For this review, take the finished solid that the model builds, in its own axes (mm). A direction names the side the tool comes from. Round coordinates to 2 decimals unless told otherwise and drop trailing zeros. Order: outer loops, then holes, each group sorted by start corner. A loop starts at its lowest first (then second) coordinate and runs counter-clockwise, first axis right, second up. Notation, with made-up numbers: M 25.25,21.5 L 76.25,21.5 A23 ccw 76.25,33.5 Z; hole C 34,61 d3. An arc over 180 degrees is marked long. Answer as a JSON object with one key per item and string values.
from build123d import *

# Parameters (mm, degrees)
SKETCH1_W                 = 71
SKETCH1_H                 = 250
BOSS_EXTRUDE1_DEPTH       = 5
SKETCH2_W                 = 65
SKETCH2_H                 = 45
BOSS_EXTRUDE3_DEPTH       = 2
LPATTERN1_COUNT           = 5
LPATTERN1_PITCH           = 50
SKETCH3_W                 = 69
SKETCH3_H                 = 48.754858224
BOSS_EXTRUDE8_DEPTH       = 25
LPATTERN5_COUNT           = 5
LPATTERN5_PITCH           = 50
LPATTERN6_COUNT           = 2
LPATTERN6_PITCH           = 70
LPATTERN6_COPY_1_SKETCH_W = 65
LPATTERN6_COPY_1_SKETCH_H = 45
LPATTERN6_COPY_1_DEPTH    = 2
LPATTERN6_COPY_2_SKETCH_W = 65
LPATTERN6_COPY_2_SKETCH_H = 45
LPATTERN6_COPY_2_DEPTH    = 2
LPATTERN6_COPY_3_SKETCH_W = 65
LPATTERN6_COPY_3_SKETCH_H = 45
LPATTERN6_COPY_3_DEPTH    = 2
LPATTERN6_COPY_4_SKETCH_W = 65
LPATTERN6_COPY_4_SKETCH_H = 45
LPATTERN6_COPY_4_DEPTH    = 2
LPATTERN6_COPY_5_SKETCH_W = 69
LPATTERN6_COPY_5_SKETCH_H = 48.754858224
LPATTERN6_COPY_5_DEPTH    = 25
LPATTERN6_COPY_6_SKETCH_W = 69
LPATTERN6_COPY_6_SKETCH_H = 48.754858224
LPATTERN6_COPY_6_DEPTH    = 25
LPATTERN6_COPY_7_SKETCH_W = 69
LPATTERN6_COPY_7_SKETCH_H = 48.754858224
LPATTERN6_COPY_7_DEPTH    = 25
LPATTERN6_COPY_8_SKETCH_W = 69
LPATTERN6_COPY_8_SKETCH_H = 48.754858224
LPATTERN6_COPY_8_DEPTH    = 25


with BuildPart() as part:
    # Sketch1 → Boss-Extrude1 (new body)
    with BuildSketch(Plane(origin=(0, 0, 0), x_dir=(1, 0, 0), z_dir=(0, 1, 0))):
        Rectangle(SKETCH1_W, SKETCH1_H)
    boss_extrude1 = extrude(amount=BOSS_EXTRUDE1_DEPTH)

    # Sketch2 → Boss-Extrude3 (add)
    with BuildSketch(Plane(origin=(0, 5, 0), x_dir=(1, 0, 0), z_dir=(0, 1, 0))):
        with Locations((0, -100)):
            Rectangle(SKETCH2_W, SKETCH2_H)
    boss_extrude3 = extrude(amount=BOSS_EXTRUDE3_DEPTH)

    # LPattern1: Boss-Extrude3 ×5
    with Locations(*[(0, 0, -i * LPATTERN1_PITCH) for i in range(1, LPATTERN1_COUNT)]):
        add(boss_extrude3)

    # Sketch3 → Boss-Extrude8 (add)
    with BuildSketch(Plane(origin=(0, 7, 0), x_dir=(1, 0, 0), z_dir=(0, 1, 0))):
        with Locations((0, -99.635002086)):
            Rectangle(SKETCH3_W, SKETCH3_H)
    boss_extrude8 = extrude(amount=BOSS_EXTRUDE8_DEPTH)

    # LPattern5: Boss-Extrude8 ×5
    with Locations(*[(0, 0, -i * LPATTERN5_PITCH) for i in range(1, LPATTERN5_COUNT)]):
        add(boss_extrude8)

    # LPattern6: Boss-Extrude1, Boss-Extrude3, Boss-Extrude8 ×2
    with Locations(*[(i * LPATTERN6_PITCH, 0, 0) for i in range(1, LPATTERN6_COUNT)]):
        add(boss_extrude1)
        add(boss_extrude3)
        add(boss_extrude8)

    # LPattern6 copy 1 sketch → LPattern6 copy 1 (add)
    with BuildSketch(Plane(origin=(70, 5, -50), x_dir=(1, 0, 0), z_dir=(0, 1, 0))):
        with Locations((0, -100)):
            Rectangle(LPATTERN6_COPY_1_SKETCH_W, LPATTERN6_COPY_1_SKETCH_H)
    extrude(amount=LPATTERN6_COPY_1_DEPTH)

    # LPattern6 copy 2 sketch → LPattern6 copy 2 (add)
    with BuildSketch(Plane(origin=(70, 5, -100), x_dir=(1, 0, 0), z_dir=(0, 1, 0))):
        with Locations((0, -100)):
            Rectangle(LPATTERN6_COPY_2_SKETCH_W, LPATTERN6_COPY_2_SKETCH_H)
    extrude(amount=LPATTERN6_COPY_2_DEPTH)

    # LPattern6 copy 3 sketch → LPattern6 copy 3 (add)
    with BuildSketch(Plane(origin=(70, 5, -150), x_dir=(1, 0, 0), z_dir=(0, 1, 0))):
        with Locations((0, -100)):
            Rectangle(LPATTERN6_COPY_3_SKETCH_W, LPATTERN6_COPY_3_SKETCH_H)
    extrude(amount=LPATTERN6_COPY_3_DEPTH)

    # LPattern6 copy 4 sketch → LPattern6 copy 4 (add)
    with BuildSketch(Plane(origin=(70, 5, -200), x_dir=(1, 0, 0), z_dir=(0, 1, 0))):
        with Locations((0, -100)):
            Rectangle(LPATTERN6_COPY_4_SKETCH_W, LPATTERN6_COPY_4_SKETCH_H)
    extrude(amount=LPATTERN6_COPY_4_DEPTH)

    # LPattern6 copy 5 sketch → LPattern6 copy 5 (add)
    with BuildSketch(Plane(origin=(70, 7, -50), x_dir=(1, 0, 0), z_dir=(0, 1, 0))):
        with Locations((0, -99.635002086)):
            Rectangle(LPATTERN6_COPY_5_SKETCH_W, LPATTERN6_COPY_5_SKETCH_H)
    extrude(amount=LPATTERN6_COPY_5_DEPTH)

    # LPattern6 copy 6 sketch → LPattern6 copy 6 (add)
    with BuildSketch(Plane(origin=(70, 7, -100), x_dir=(1, 0, 0), z_dir=(0, 1, 0))):
        with Locations((0, -99.635002086)):
            Rectangle(LPATTERN6_COPY_6_SKETCH_W, LPATTERN6_COPY_6_SKETCH_H)
    extrude(amount=LPATTERN6_COPY_6_DEPTH)

    # LPattern6 copy 7 sketch → LPattern6 copy 7 (add)
    with BuildSketch(Plane(origin=(70, 7, -150), x_dir=(1, 0, 0), z_dir=(0, 1, 0))):
        with Locations((0, -99.635002086)):
            Rectangle(LPATTERN6_COPY_7_SKETCH_W, LPATTERN6_COPY_7_SKETCH_H)
    extrude(amount=LPATTERN6_COPY_7_DEPTH)

    # LPattern6 copy 8 sketch → LPattern6 copy 8 (add)
    with BuildSketch(Plane(origin=(70, 7, -200), x_dir=(1, 0, 0), z_dir=(0, 1, 0))):
        with Locations((0, -99.635002086)):
            Rectangle(LPATTERN6_COPY_8_SKETCH_W, LPATTERN6_COPY_8_SKETCH_H)
    extrude(amount=LPATTERN6_COPY_8_DEPTH)


solid = part.part
1) Insertion check: P1, Ø12, axis at y = 20, z = 23.5, coming from the -X side; P2, Ø0.6, axis at y = 6, z = -43.5, coming from the -X side; P3, Ø6, axis at y = 21, z = -73.5, coming from the +X side. Each pin has a flat end and moves straight along its axis. Give the tip position at first contact, or say it passes through.
Geometry check:
{"P1": "stops at x = -34.5", "P2": "stops at x = -32.5", "P3": "stops at x = 104.5"}
2) Mouldability with a two-part tool opening along Z and no side actions: class faces 1 (the flat face through (-3, 7, 23)), 2 (the flat face through (0, 32, 49)), 3 (the flat face through (34, 2, -125)) as +Z half, -Z half, draft (parallel to the pull), parting line (faces both ways), or undercut.
Geometry check:
{"face 1": "undercut", "face 2": "draft", "face 3": "-Z half"}
3) Machinability: for faces 4 (the flat face through (35.5, 19, 0)), 5 (the flat face through (70, 19, 74.012)), 6 (the flat face through (67, 7, -27)), 7 (the flat face through (0, 19, -124.742)), which of the approach directions +Z, -Z, +X, -X, +Y, -Y give a long, thin tool a straight path to every point of the face, cutting with its end or side? Answer none if there is none.
Geometry check:
{"face 4": "+Z, -Z, +Y", "face 5": "+X, -X, +Y", "face 6": "none", "face 7": "-Z, +X, -X, +Y"}
4) Add section A-A on z = -61. State the section outline as (x, y) points.
Geometry check:
{"outline": "M -35.5,0 L 105.5,0 L 105.5,5 L 102.5,5 L 102.5,7 L 104.5,7 L 104.5,32 L 35.5,32 L 35.5,7 L 37.5,7 L 37.5,5 L 32.5,5 L 32.5,7 L 34.5,7 L 34.5,32 L -34.5,32 L -34.5,7 L -32.5,7 L -32.5,5 L -35.5,5 Z"}
5) Add section B-B on y = 21. State how many separate pieces and enclosed holes the cut face has, and give its area (3 significant figures).
Geometry check:
{"separate pieces": "10", "enclosed holes": "0", "area": "33,600 mm²"}
6) For L1, parallel to Z at x = 63.5, y = 7.5; L2, parallel to X at y = 22, z = -21, list the stretches that pass through material, from the lowest coordinate up.
Geometry check:
{"L1": "z = -124.74 to -75.99, -74.74 to -25.99, -24.74 to 24.01, 25.26 to 74.01, 75.26 to 124.01", "L2": "x = -34.5 to 34.5, 35.5 to 104.5"}
